```python
from build123d import *

# Parameters (mm, degrees)
SKETCH1_W                   = 90
SKETCH1_H                   = 90
BOSS_EXTRUDE1_DEPTH         = 8
FILLET1_R                   = 10
SKETCH2_R                   = 45
BOSS_EXTRUDE2_DEPTH         = 137
SKETCH3_R                   = 8.5
BOSS_EXTRUDE3_DEPTH         = 32
F_6_0_MM_DOWEL_HOLES1_D     = 6
F_6_0_MM_DOWEL_HOLES1_DEPTH = 30
F_6_0_MM_DOWEL_HOLES1_TIP   = 1.802581857
SKETCH8_W                   = 90
SKETCH8_H                   = 90
BOSS_EXTRUDE4_DEPTH         = 32
CHAMFER2_SIZE               = 20
FILLET2_R                   = 10


with BuildPart() as part:
    # Sketch1 → Boss-Extrude1 (new body)
    with BuildSketch(Plane.XY):
        Rectangle(SKETCH1_W, SKETCH1_H)
    extrude(amount=BOSS_EXTRUDE1_DEPTH)

    # Fillet1
    fillet1_edges = [part.edges().sort_by_distance(p)[0] for p in [
        (-45, 45, 4),
        (45, 45, 4),
        (45, -45, 4),
        (-45, -45, 4),
    ]]
    fillet(fillet1_edges, radius=FILLET1_R)

    # Sketch2 → Boss-Extrude2 (add)
    with BuildSketch(Plane.XY.offset(8)):
        Circle(SKETCH2_R)
    extrude(amount=-BOSS_EXTRUDE2_DEPTH)

    # Sketch3 → Boss-Extrude3 (add)
    with BuildSketch(Plane.XY.offset(8)):
        Circle(SKETCH3_R)
    extrude(amount=BOSS_EXTRUDE3_DEPTH)

    # Ø6.0 mm Dowel Holes1
    with Locations(Plane.XY.offset(8)):
        with Locations((-35, 35), (35, 35), (35, -35), (-35, -35)):
            Hole(F_6_0_MM_DOWEL_HOLES1_D / 2, depth=F_6_0_MM_DOWEL_HOLES1_DEPTH)
            with Locations((0, 0, -(F_6_0_MM_DOWEL_HOLES1_DEPTH + F_6_0_MM_DOWEL_HOLES1_TIP / 2))):  # 118° drill point
                Cone(0, F_6_0_MM_DOWEL_HOLES1_D / 2, F_6_0_MM_DOWEL_HOLES1_TIP, mode=Mode.SUBTRACT)

    # Sketch8 → Boss-Extrude4 (add)
    with BuildSketch(Plane(origin=(0, 0, -129), x_dir=(-1, 0, 0), z_dir=(0, 0, -1))):
        Rectangle(SKETCH8_W, SKETCH8_H)
    extrude(amount=-BOSS_EXTRUDE4_DEPTH)

    # Chamfer2
    chamfer2_edges = [part.edges().sort_by_distance(p)[0] for p in [
        (45, -45, -113),
        (45, 45, -113),
        (-45, 45, -113),
        (-45, -45, -113),
    ]]
    chamfer(chamfer2_edges, length=CHAMFER2_SIZE)

    # Fillet2
    fillet2_edges = [part.edges().sort_by_distance(p)[0] for p in [
        (45, 0, -129),
        (45, 25, -113),
        (45, -25, -113),
        (-45, 0, -129),
        (0, 45, -129),
        (0, -45, -129),
        (35, 35, -129),
        (-35, 35, -129),
        (-35, -35, -129),
        (35, -35, -129),
        (-25, -45, -113),
        (25, -45, -113),
        (-45, 25, -113),
        (-45, -25, -113),
        (25, 45, -113),
        (-25, 45, -113),
    ]]
    fillet(fillet2_edges, radius=FILLET2_R)


solid = part.part
```
Read the model definition and answer for the solid it produces. Units are mm, in the model's axes. A direction names the side the tool comes from. Coordinates: 2 decimals unless noted, no trailing zeros. Write each loop counter-clockwise with the first axis right and the second up, starting at its lowest first coordinate (ties: lowest second). Pieces come first, ordered by that corner, then holes. Notation, with made-up numbers: (47, -20.75) -> (82, -20.75) arc R9 ccw to (82, -4.75) -> close; hole circle Ø2 at (-20.5, 47.25). An arc over 180 degrees is marked (long way). Answer as a JSON object with one key per item and string values.
Q1. A tool of negligible diameter and unlimited length cuts with its end or side. For faces 1 (the cylindrical face through (44.26, 24.63, -107.85)), 2 (the cylindrical face through (4.57, 7.167, 23.776)), 3 (the flat face through (35, -35, -108)), from which of +Z, -Z, +X, -X, +Y, -Y can it reach the whole face along a straight path? Write none if from no direction.
The answers:
{"face 1": "-Z, +X, +Y", "face 2": "+Z", "face 3": "-Z, +X, -Y"}
Q2. Determine the mould class of faces 4 (the cylindrical face through (0.29, 41.99, -126.15)), 5 (the cylindrical face through (24.735, -44.218, -107.846)), 6 (the cylindrical face through (37.21, 37.03, 3.94)), 7 (the flat face through (-32, 33, -97)) for opening direction Y: pulls with the +Y half, pulls with the -Y half, needs draft (parallel to the pull), parting line crosses it, or undercut.
The answers:
{"face 4": "pulls with the +Y half", "face 5": "pulls with the -Y half", "face 6": "undercut", "face 7": "needs draft"}
Q3. The part is cut by section A-A on z = -112. Give the vertices of the cut face in (x, y), then the cut area to 3 significant figures.
The answers:
{"outline": "(-45, -20.86) arc R10 ccw to (-42.07, -27.93) -> (-27.93, -42.07) arc R10 ccw to (-20.86, -45) -> (20.86, -45) arc R10 ccw to (27.93, -42.07) -> (42.07, -27.93) arc R10 ccw to (45, -20.86) -> (45, 20.86) arc R10 ccw to (42.07, 27.93) -> (27.93, 42.07) arc R10 ccw to (20.86, 45) -> (-20.86, 45) arc R10 ccw to (-27.93, 42.07) -> (-42.07, 27.93) arc R10 ccw to (-45, 20.86) -> close", "area": "7,280 mm2"}
Q4. The part is cut by section C-C on x = 15. Give the vertices of the cut face in (y, z).
The answers:
{"outline": "(-45, -119) arc R10 ccw to (-35, -129) -> (35, -129) arc R10 ccw to (45, -119) -> (45, -97) -> (42.43, -97) -> (42.43, 0) -> (45, 0) -> (45, 8) -> (-45, 8) -> (-45, 0) -> (-42.43, 0) -> (-42.43, -97) -> (-45, -97) -> close"}
Q5. The part is cut by section B-B on y = -4. Give the vertices of the cut face in (x, z), then the cut area to 3 significant figures.
The answers:
{"outline": "(-45, -119) arc R10 ccw to (-35, -129) -> (35, -129) arc R10 ccw to (45, -119) -> (45, -97) -> (44.82, -97) -> (44.82, 0) -> (45, 0) -> (45, 8) -> (7.5, 8) -> (7.5, 40) -> (-7.5, 40) -> (-7.5, 8) -> (-45, 8) -> (-45, 0) -> (-44.82, 0) -> (-44.82, -97) -> (-45, -97) -> close", "area": "12,700 mm2"}
Q6. Consider line 1 (Y direction, x = 35, z = 3.5); line 2 (Z direction, x = 18, y = 2); line 3 (Y direction, x = -6.5, z = -85.5). Determine where each line is inside the solid, lowest interval first. Write a range as [from, to].
The answers:
{"line 1": "y = [-45, -38], [-32, 32], [38, 45]", "line 2": "z = [-129, 8]", "line 3": "y = [-44.53, 44.53]"}
Q7. Flat-ended cylindrical pins translate along their axes: pin 1 Ø1 at (x, z) = (-26.5, -50) entering from -Y; pin 2 Ø12 at (y, z) = (-10.5, -28.5) entering from +X; pin 3 Ø8 at (x, y) = (-35, -35) entering from -Z. Find the tip coordinate at first contact, or state that the pin passes through.
The answers:
{"pin 1": "stops at y = -36.73", "pin 2": "stops at x = 44.77", "pin 3": "stops at z = -127"}
Q8. The part is cut by section D-D on z = -48.5. Give the vertices of the cut face in (x, y).
The answers:
{"outline": "circle Ø90 at (0, 0)"}
